from build123d import *

# Parameters (mm, degrees)
SKETCH_1_W          = 40
SKETCH_1_H          = 26
EXTRUDE_1_DEPTH     = 35
CUT_EXTRUDE_1_DEPTH = 43.355637169
SKETCH_4_R          = 2.5
CUT_EXTRUDE_2_DEPTH = 46.453272709
CUT_EXTRUDE_3_DEPTH = 43.355637169
SKETCH_7_W          = 8
SKETCH_7_H          = 2
CUT_EXTRUDE_4_DEPTH = 43.355637169
CHAMFER_1_SIZE      = 1
EXTRUDE_START       = -21
SKETCH_9_R          = 2.5
EXTRUDE_2_DEPTH     = 21
SKETCH_10_R         = 2.7
CUT_EXTRUDE_5_DEPTH = 48.968739821
SKETCH_13_R         = 2.5
EXTRUDE_3_DEPTH     = 21
SKETCH_14_R         = 2.7
CUT_EXTRUDE_6_DEPTH = 48.968739821
SKETCH_15_R         = 2.7
CUT_EXTRUDE_7_DEPTH = 48.968739821


with BuildPart() as part:
    # Эскиз1 → Бобышка-Вытянуть1 (new body)
    with BuildSketch(Plane.XY):
        Rectangle(SKETCH_1_W, SKETCH_1_H)
    extrude(amount=EXTRUDE_1_DEPTH)

    # Эскиз2 → Вырез-Вытянуть1 (cut, through all)
    with BuildSketch(Plane(origin=(0, 0, 0), x_dir=(-1, 0, 0), z_dir=(0, 0, -1))):
        Polygon((-10, 8), (-5, 13), (-20, 13), (-20, 8), align=None)
        Polygon((20, 13), (5, 13), (10, 8), (20, 8), align=None)
        with BuildLine():
            ThreePointArc((5, 0), (3.535533906, 3.535533906), (0, 5))
            Line((0, 5), (0, 0))
            Line((0, 0), (0, -5))
            ThreePointArc((0, -5), (3.535533906, -3.535533906), (5, 0))
        make_face()
        with BuildLine():
            Line((0, 0), (0, 5))
            ThreePointArc((0, 5), (-5, 0), (0, -5))
            Line((0, -5), (0, 0))
        make_face()
    extrude(amount=-CUT_EXTRUDE_1_DEPTH, mode=Mode.SUBTRACT)

    # Эскиз4 → Вырез-Вытянуть2 (cut, through all)
    with BuildSketch(Plane(origin=(0, 8, 0), x_dir=(1, 0, 0), z_dir=(0, 1, 0))):
        with BuildLine():
            ThreePointArc((-12.5, -7), (-15, -4.5), (-17.5, -7))
            Line((-17.5, -7), (-12.5, -7))
        make_face()
        with BuildLine():
            Line((-12.5, -7), (-17.5, -7))
            ThreePointArc((-17.5, -7), (-15, -9.5), (-12.5, -7))
        make_face()
        with BuildLine():
            ThreePointArc((-12.5, -28), (-15, -25.5), (-17.5, -28))
            Line((-17.5, -28), (-12.5, -28))
        make_face()
        with BuildLine():
            Line((-12.5, -28), (-17.5, -28))
            ThreePointArc((-17.5, -28), (-15, -30.5), (-12.5, -28))
        make_face()
        with Locations(Location((15, -28, 0), (0, 0, 180))):
            Circle(SKETCH_4_R)
        with Locations(Location((15, -7, 0), (0, 0, 180))):
            Circle(SKETCH_4_R)
    extrude(amount=-CUT_EXTRUDE_2_DEPTH, mode=Mode.SUBTRACT)

    # Эскиз6 → Вырез-Вытянуть3 (cut, through all)
    with BuildSketch(Plane.XY.offset(35)):
        Polygon((-18.878222765, 8), (-20, 8), (-20, -5), (-18.878222765, -4), align=None)
        Polygon((18.878222765, 8), (18.878222765, -4), (20, -5), (20, 8), align=None)
    extrude(amount=-CUT_EXTRUDE_3_DEPTH, mode=Mode.SUBTRACT)

    # Эскиз7 → Вырез-Вытянуть4 (cut, through all)
    with BuildSketch(Plane.XY.offset(35)):
        with Locations((-4, -12)):
            Rectangle(SKETCH_7_W, SKETCH_7_H)
        with Locations((4, -12)):
            Rectangle(SKETCH_7_W, SKETCH_7_H)
    extrude(amount=-CUT_EXTRUDE_4_DEPTH, mode=Mode.SUBTRACT)

    # Фаска1
    chamfer_1_edges = [part.edges().sort_by_distance(p)[0] for p in [
        (20, -13, 17.5),
        (-20, -13, 17.5),
        (8, -13, 17.5),
        (-8, -13, 17.5),
    ]]
    chamfer(chamfer_1_edges, length=CHAMFER_1_SIZE)

    # Эскиз9 → Бобышка-Вытянуть2 (add)
    with BuildSketch(Plane.XZ.offset(13).offset(EXTRUDE_START)):
        with Locations((-15, 28)):
            Circle(SKETCH_9_R)
    extrude(amount=EXTRUDE_2_DEPTH)

    # Эскиз10 → Вырез-Вытянуть5 (cut, through all)
    with BuildSketch(Plane.XZ.offset(13)):
        with Locations(Location((-14, 28, 0), (0, 0, 270))):
            Circle(SKETCH_10_R)
    extrude(amount=-CUT_EXTRUDE_5_DEPTH, mode=Mode.SUBTRACT)

    # Эскиз13 → Бобышка-Вытянуть3 (add)
    with BuildSketch(Plane.XZ.offset(13).offset(EXTRUDE_START)):
        with Locations((-15, 7)):
            Circle(SKETCH_13_R)
        with Locations((15, 7)):
            Circle(SKETCH_13_R)
        with Locations((15, 28)):
            Circle(SKETCH_13_R)
    extrude(amount=EXTRUDE_3_DEPTH)

    # Эскиз14 → Вырез-Вытянуть6 (cut, through all)
    with BuildSketch(Plane.XZ.offset(13)):
        with Locations(Location((14, 28, 0), (0, 0, 270))):
            Circle(SKETCH_14_R)
    extrude(amount=-CUT_EXTRUDE_6_DEPTH, mode=Mode.SUBTRACT)

    # Эскиз15 → Вырез-Вытянуть7 (cut, through all)
    with BuildSketch(Plane.XZ.offset(13)):
        with Locations(Location((-14, 7, 0), (0, 0, 270))):
            Circle(SKETCH_15_R)
        with Locations(Location((14, 7, 0), (0, 0, 270))):
            Circle(SKETCH_15_R)
    extrude(amount=-CUT_EXTRUDE_7_DEPTH, mode=Mode.SUBTRACT)


solid = part.part
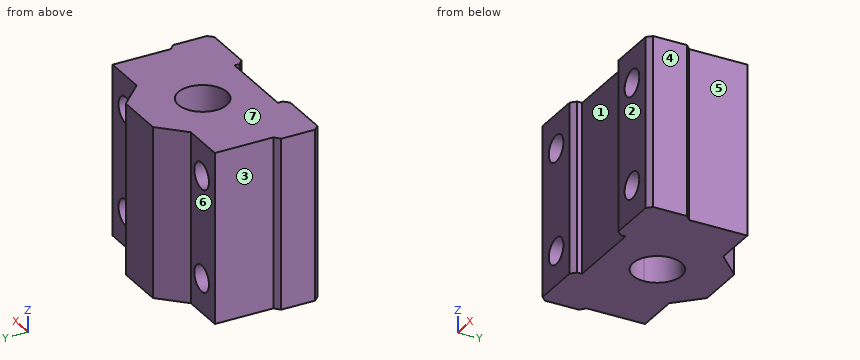
Can you work these out from the model? Positions are in its coordinate system, mm. Face numbers are marked on the shaded views. A direction names the side the tool comes from. Round coordinates to 2 decimals unless told otherwise and drop trailing zeros. Loops run counter-clockwise (first coordinate to the right, second up) from the corner with the lowest first, then second, coordinate; pieces in that order, holes last. Notation, with made-up numbers: (23.5, -39.75) - (55.5, -39.75) arc R20 cw to (55.5, -17.75) - close; hole circle Ø10 at (73.5, 80.25). An arc over 180 degrees is marked (long way). Use CSV: the item, a comma, the result in double quotes. Start each with the question number.
1) We'd pull the mould along X, two halves only. Please class the marked faces 1, 2, 3 and 4: released by +X, released by -X, zero draft, split by the parting line, or undercut.
2) If we section it at A-A on y = 4: Write out the boundary of the cut face in (x, z).
3) Please list where these lines run through material, in increasing order: probe 1 along X at (y, z) = (-0.5, 7); probe 2 along X at (y, z) = (0.75, 28); probe 3 along X at (y, z) = (-5.5, 7). Write a range as [from, to].
4) For the marked faces 5, 6 and 7, which set-ups out of +Z, -Z, +X, -X, +Y, -Y let a thin tool reach every point of the face, with its end or its side?
5) If we section it at D-D on y = -8: Write out the boundary of the cut face in (x, z).
6) If we section it at C-C on x = 4: Write out the boundary of the cut face in (y, z), plus the area to 3 significant figures.
7) If we section it at B-B on z = 7: Count the separate pieces of the cut face and the enclosed holes in it, plus the area to 3 significant figures.
8) For pin 1 Ø12 at (x, z) = (1.5, 23.5) entering from -Y; pin 2 Ø9.5 at (y, z) = (0.5, 19.5) entering from -X; pin 3 Ø2.5 at (x, z) = (-15.5, 9) entering from +Y, each with a flat end and sliding along its axis, tell me the tip position at first contact or that it passes through.
Geometry results:
1,face 1,"undercut"
1,face 2,"zero draft"
1,face 3,"released by -X"
1,face 4,"released by +X"
2,outline,"(-18.88, 0) - (-3, 0) - (-3, 35) - (-18.88, 35) - close; (3, 0) - (18.88, 0) - (18.88, 35) - (3, 35) - close; hole circle Ø5.4 at (-14, 7); hole circle Ø5.4 at (-14, 28); hole circle Ø5.4 at (14, 7); hole circle Ø5.4 at (14, 28)"
3,probe 1,"x = [-18.88, -16.7], [-11.3, -4.97], [4.97, 11.3], [16.7, 18.88]"
3,probe 2,"x = [-18.88, -16.7], [-11.3, -4.94], [4.94, 11.3], [16.7, 18.88]"
3,probe 3,"x = [-20, -16.7], [-11.3, 11.3], [16.7, 20]"
4,face 5,"+Z, -Z, +X, +Y"
4,face 6,"+Z, -Z, -X, +Y"
4,face 7,"+Z, +X, -X, +Y, -Y"
5,outline,"(-20, 0) - (20, 0) - (20, 35) - (-20, 35) - close; hole circle Ø5.4 at (-14, 7); hole circle Ø5.4 at (-14, 28); hole circle Ø5.4 at (14, 7); hole circle Ø5.4 at (14, 28)"
6,outline,"(-11, 0) - (-3, 0) - (-3, 35) - (-11, 35) - close; (3, 0) - (13, 0) - (13, 35) - (3, 35) - close"
6,area,"630 mm2"
7,separate pieces,"3"
7,enclosed holes,"1"
7,area,"548 mm2"
8,pin 1,"stops at y = -11"
8,pin 2,"stops at x = -19.16"
8,pin 3,"stops at y = 8"
